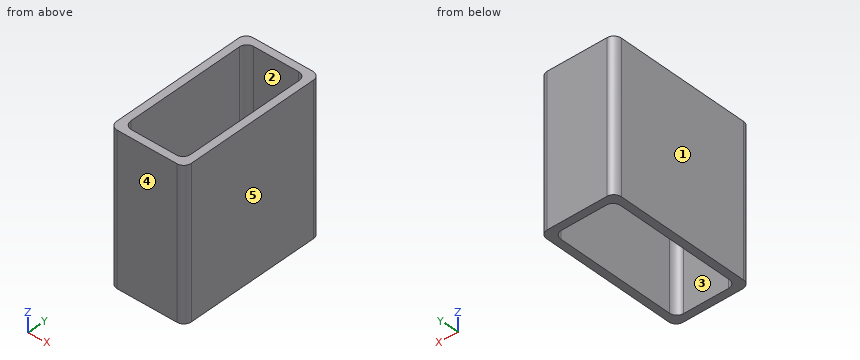
from build123d import *

# Parameters (mm, degrees)
SZKIC1_W                    = 24
SZKIC1_H                    = 54
DODANIE_WYCI_GNI_CIE1_DEPTH = 60
ZAOKR_GLENIE1_R             = 3


with BuildPart() as part:
    # Szkic1 → Dodanie-wyciągnięcie1 (new body)
    with BuildSketch(Plane.XY):
        with BuildLine():
            Line((-12, -30), (12, -30))
            ThreePointArc((12, -30), (14.121320344, -29.121320344), (15, -27))
            Line((15, -27), (15, 27))
            ThreePointArc((15, 27), (14.121320344, 29.121320344), (12, 30))
            Line((12, 30), (-12, 30))
            ThreePointArc((-12, 30), (-14.121320344, 29.121320344), (-15, 27))
            Line((-15, 27), (-15, -27))
            ThreePointArc((-15, -27), (-14.121320344, -29.121320344), (-12, -30))
        make_face()
        Rectangle(SZKIC1_W, SZKIC1_H, mode=Mode.SUBTRACT)
    extrude(amount=DODANIE_WYCI_GNI_CIE1_DEPTH)

    # Zaokrąglenie1
    zaokr_glenie1_edges = [part.edges().sort_by_distance(p)[0] for p in [
        (-12, 27, 30),
        (-12, -27, 30),
        (12, -27, 30),
        (12, 27, 30),
    ]]
    fillet(zaokr_glenie1_edges, radius=ZAOKR_GLENIE1_R)


solid = part.part
Input: part model. Units: mm. Frame: model coordinates. Face numbers are marked on the shaded views. A direction names the side the tool comes from. Give positions to 0.01 mm unless a question says otherwise; leave off trailing zeros. Order: outer loops, then holes, each group sorted by start corner. A loop starts at its lowest first (then second) coordinate and runs counter-clockwise, first axis right, second up. Notation, with made-up numbers: (41.25, 19) -> (73.25, 19) arc R5 cw to (73.25, 25) -> close; hole circle Ø9 at (76.25, -27.5). An arc over 180 degrees is marked (long way). Use one line per item in the form item = value.
1) Section C-C, the plane z = 52. Return loops of the section in (x, y), and give its area (3 significant figures).
Response values:
outline = (-15, -27) arc R3 ccw to (-12, -30) -> (12, -30) arc R3 ccw to (15, -27) -> (15, 27) arc R3 ccw to (12, 30) -> (-12, 30) arc R3 ccw to (-15, 27) -> close; hole (-12, -24) arc R3 ccw to (-9, -27) -> (9, -27) arc R3 ccw to (12, -24) -> (12, 24) arc R3 ccw to (9, 27) -> (-9, 27) arc R3 ccw to (-12, 24) -> close
area = 504 mm^2
2) Section B-B, the plane x = -4. Return loops of the section in (y, z), and give its area (3 significant figures).
Response values:
outline = (-30, 0) -> (-27, 0) -> (-27, 60) -> (-30, 60) -> close; (27, 0) -> (30, 0) -> (30, 60) -> (27, 60) -> close
area = 360 mm^2
3) Reachability of the marked faces 1 and 2 from +Z, -Z, +X, -X, +Y, -Y: full face, straight path, thin tool, end or side. Return the list, or none.
Response values:
face_1 = +Z, -Z, -X, +Y, -Y
face_2 = +Z, -Z
4) Section A-A, the plane y = 14. Return loops of the section in (x, z), and give its area (3 significant figures).
Response values:
outline = (-15, 0) -> (-12, 0) -> (-12, 60) -> (-15, 60) -> close; (12, 0) -> (15, 0) -> (15, 60) -> (12, 60) -> close
area = 360 mm^2
5) Line query: probe 1 along Y at (x, z) = (9, 9.5); probe 2 along X at (y, z) = (2.5, 12.5); probe 3 along Y at (x, z) = (-11, 42.5). Output: solid intervals per line, ascending.
Response values:
probe_1 = -30 to -27, 27 to 30
probe_2 = -15 to -12, 12 to 15
probe_3 = -30 to -26.24, 26.24 to 30
6) Mould query, pull axis Y, two halves, no side actions, for the marked faces 3, 4 and 5. Classes: pulls with the +Y half, pulls with the -Y half, needs draft (parallel to the pull), parting line crosses it, or undercut.
Response values:
face_3 = undercut
face_4 = pulls with the -Y half
face_5 = needs draft
